from build123d import *

# Parameters (mm, degrees)
BASE_FLANGE4_DEPTH           = 127
EDGE_FLANGE1_STRIP_W         = 19.05
EDGE_FLANGE1_STRIP_H         = 3.175
EDGE_FLANGE1_STRIP_CUT_DEPTH = 250.825
EDGE_FLANGE1_DEPTH           = 250.825
SKETCH28_W                   = 44.45
SKETCH28_H                   = 41.275
SKETCH28_H_2                 = 38.1
CUT_EXTRUDE1_DEPTH           = 312.085197333
F_10_32_TAPPED_HOLE1_D       = 4.0386
F_12_28_TAPPED_HOLE1_D       = 4.6228


# Sheet-metal steps are written as plain solids
with BuildPart() as part:
    # Sketch1 → Base-Flange4 (new body)
    with BuildSketch(Plane.XY):
        with BuildLine():
            Line((254, 0), (3.175, 0))
            ThreePointArc((3.175, 0), (0.92993597, 0.92993597), (0, 3.175))
            Line((0, 3.175), (0, 63.5))
            Line((0, 63.5), (-3.175, 63.5))
            Line((-3.175, 63.5), (-3.175, 3.175))
            ThreePointArc((-3.175, 3.175), (-1.315128061, -1.315128061), (3.175, -3.175))
            Line((3.175, -3.175), (254, -3.175))
            Line((254, -3.175), (254, 0))
        make_face()
    extrude(amount=BASE_FLANGE4_DEPTH)

    # Edge-Flange1 strip (across the edge) → Edge-Flange1 strip cut (cut)
    with BuildSketch(Plane.ZY.offset(-254)):
        with Locations((-6.35, -1.5875)):
            Rectangle(EDGE_FLANGE1_STRIP_W, EDGE_FLANGE1_STRIP_H)
    extrude(amount=EDGE_FLANGE1_STRIP_CUT_DEPTH, mode=Mode.SUBTRACT)

    # Edge-Flange1 section (across the edge) → Edge-Flange1 (add)
    with BuildSketch(Plane.ZY.offset(-254)):
        with BuildLine():
            Line((-3.175, 3.175), (-3.175, 123.825))
            Line((-3.175, 123.825), (0, 123.825))
            Line((0, 123.825), (0, 3.175))
            ThreePointArc((0, 3.175), (0.92993597, 0.92993597), (3.175, 0))
            Line((3.175, 0), (3.175, -3.175))
            ThreePointArc((3.175, -3.175), (-1.315128061, -1.315128061), (-3.175, 3.175))
        make_face()
    extrude(amount=EDGE_FLANGE1_DEPTH)

    # Sketch28 → Cut-Extrude1 (cut, through all)
    with BuildSketch(Plane.XZ.offset(3.175)):
        with Locations((231.775, 106.3625)):
            Rectangle(SKETCH28_W, SKETCH28_H)
        with Locations((231.775, 22.225)):
            Rectangle(SKETCH28_W, SKETCH28_H_2)
    extrude(amount=-CUT_EXTRUDE1_DEPTH, mode=Mode.SUBTRACT)

    # #10-32 Tapped Hole1 (through all)
    with Locations(Plane(origin=(0, -3.175, 0), x_dir=(-1, 0, 0), z_dir=(0, -1, 0))):
        with Locations((-222.25, -50.8), (-196.85, -50.8), (-196.85, -76.2), (-222.25, -76.2)):
            Hole(F_10_32_TAPPED_HOLE1_D / 2)

    # #12-28 Tapped Hole1 (through all)
    with Locations(Plane(origin=(0, 0, 0), x_dir=(0, 0, -1), z_dir=(1, 0, 0))):
        with Locations((-12.7, 50.8), (-12.7, 12.7), (-114.3, 12.7), (-114.3, 50.8)):
            Hole(F_12_28_TAPPED_HOLE1_D / 2)


solid = part.part
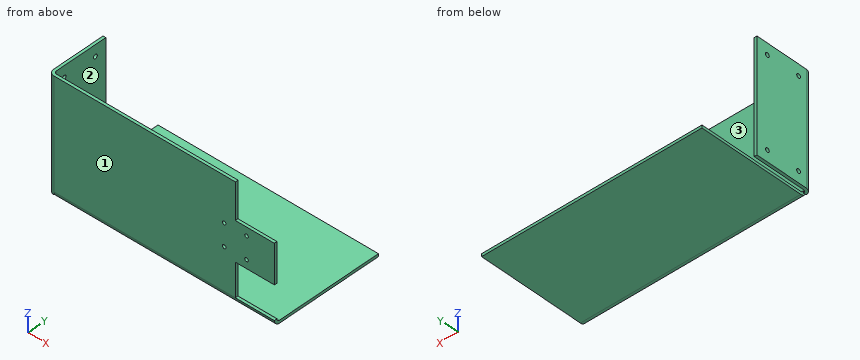
Input: part model. Units: mm. Frame: model coordinates. Face numbers are marked on the shaded views. A direction names the side the tool comes from. Give positions to 0.01 mm unless a question says otherwise; leave off trailing zeros. Loops run counter-clockwise (first coordinate to the right, second up) from the corner with the lowest first, then second, coordinate; pieces in that order, holes last. Notation, with made-up numbers: (33.5, -20) -> (50.5, -20) arc R14 cw to (50.5, -12) -> close; hole circle Ø2 at (5.25, 18.25). An arc over 180 degrees is marked (long way). Answer as a JSON object with one key per item and string values. Group by question number.
Item 1: Reachability of the marked faces 1, 2 and 3 from +Z, -Z, +X, -X, +Y, -Y: full face, straight path, thin tool, end or side. Return the list, or none.
Item 2: Cut plane B-B, the plane y = 41. Return the cut outline in (x, z) (3 decimals), and give its area (3 significant figures).
Item 3: Cut plane D-D, the plane x = 84. Return the cut outline in (y, z) (3 decimals), and give its area (3 significant figures).
Item 4: Cut plane C-C, the plane z = 67. Return the cut outline in (x, y) (3 decimals).
Item 5: Line query: probe 1 along Y at (x, z) = (-1.6, 12.7); probe 2 along Z at (x, y) = (222.25, -1.35) (3 decimals); probe 3 along Z at (x, y) = (-1, 50). Output: solid intervals per line, ascending.
Item 6: Pin query (flat end, axial travel): P1, Ø3, axis at x = 97, z = 67.5, coming from the +Y side; P2, Ø7.5, axis at y = 12.7, z = 12.7, coming from the +X side; P3, Ø1.5, axis at x = 37, y = 107, coming from the +Z side; P4, Ø5.5, axis at y = 12.7, z = 114.3, coming from the -X side (3 decimals). Return the tip coordinate at first contact, or that it passes through.
Item 7: Cut plane A-A, the plane x = 216. Return the cut outline in (y, z) (3 decimals), and give its area (3 significant figures).
Checks:
{
 "1": {"face 1": "+Z, -Z, +X, -X, -Y", "face 2": "+Z, -Z, +X, +Y", "face 3": "+Z, +X, +Y"},
 "2": {"outline": "(-3.175, 0) -> (0, 0) -> (0, 127) -> (-3.175, 127) -> close; (3.175, -3.175) -> (254, -3.175) -> (254, 0) -> (3.175, 0) -> close", "area": "1,200 mm²"},
 "3": {"outline": "(-3.175, 3.175) arc R6.35 ccw to (3.175, -3.175) -> (123.825, -3.175) -> (123.825, 0) -> (3.175, 0) arc R3.175 cw to (0, 3.175) -> (0, 127) -> (-3.175, 127) -> close", "area": "800 mm²"},
 "4": {"outline": "(-3.175, 3.175) arc R6.35 ccw to (3.175, -3.175) -> (254, -3.175) -> (254, 0) -> (3.175, 0) arc R3.175 cw to (0, 3.175) -> (0, 63.5) -> (-3.175, 63.5) -> close"},
 "5": {"probe 1": "y = -1.01 to 10.39, 15.01 to 48.49, 53.11 to 63.5", "probe 2": "z = -1.28 to 3.175, 41.275 to 48.781, 52.819 to 74.181, 78.219 to 85.725", "probe 3": "z = 0 to 10.53, 14.87 to 112.13, 116.47 to 127"},
 "6": {"P1": "stops at y = 0", "P2": "stops at x = 0", "P3": "stops at z = 0", "P4": "stops at x = -3.175"},
 "7": {"outline": "(-3.175, 3.175) arc R6.35 ccw to (3.175, -3.175) -> (123.825, -3.175) -> (123.825, 0) -> (3.175, 0) arc R3.175 cw to (0, 3.175) -> close; (-3.175, 41.275) -> (0, 41.275) -> (0, 85.725) -> (-3.175, 85.725) -> close", "area": "548 mm²"}
}
